```python
from build123d import *

# Parameters (mm, degrees)
F0_W     = 55.8
F0_H     = 27.9
F0_R     = 1.5
F0_R_2   = 3
F1_DEPTH = 4
F2_R     = 13.94999


# Not quite as in the source:
# - a fillet or chamfer is up to 0.001 mm smaller than in the source, because OpenCascade refuses the exact size


with BuildPart() as f1:
    # F0 (on Top) → F1 (new body)
    with BuildSketch(Plane.XY):
        with Locations((-27.9, 13.95)):
            Rectangle(F0_W, F0_H)
        with Locations((-19.6068542495, 8.2931457505)):
            Circle(F0_R, mode=Mode.SUBTRACT)
        with Locations((-7.2324855787, 7.2324855787)):
            Circle(F0_R, mode=Mode.SUBTRACT)
        with Locations((-20.6675144213, 20.6675144213)):
            Circle(F0_R, mode=Mode.SUBTRACT)
        with Locations((-13.95, 13.95)):
            Circle(F0_R_2, mode=Mode.SUBTRACT)
        with Locations((-8.2931457505, 19.6068542495)):
            Circle(F0_R, mode=Mode.SUBTRACT)
    extrude(amount=F1_DEPTH)

    # F2 (radius 13.95 in the source; OpenCascade refuses exactly that, so slightly less here)
    f2_edges = [f1.edges().sort_by_distance(p)[0] for p in [
        (0, 27.9, 2),
        (0, 0, 2),
    ]]
    fillet(f2_edges, radius=F2_R)


solid = f1.part
```
Geometry: final body of the model. Coordinates: model frame, mm. Coordinates: 2 decimals unless noted, no trailing zeros. Order: outer loops, then holes, each group sorted by start corner. A loop starts at its lowest first (then second) coordinate and runs counter-clockwise, first axis right, second up. Notation, with made-up numbers: (55, 14) - (109, 14) arc R19 ccw to (109, 42) - close; hole circle Ø2 at (31.25, -1.5). An arc over 180 degrees is marked (long way). Return JSON: item names as keys, results as strings. Group by question number.
1. Pull-direction query (X, two-part tool) for faces 1 (the face through (-35, 27.9, 2)), 2 (the face through (-55.8, 14, 2)), 3 (the face through (-22.166, 20.733, 1.972)), 4 (the face through (-4.195, 23.922, 2.028)); classes: pulls with the +X half, pulls with the -X half, needs draft (parallel to the pull), parting line crosses it, or undercut.
2. Pin query (flat end, axial travel): pin 1 (2 mm diameter, centred on x = -9.5, z = 0.5, fed in from -Y). Return the tip coordinate at first contact, or that it passes through.
3. Material intervals for line 1 along X through (y, z) = (20.75, 2.3); line 2 along Y through (x, z) = (-13.95, 2.45); line 3 along X through (y, z) = (12, 3.25), sorted ascending. Write a range as [from, to].
4. Cut plane B-B (y = 16). Output: boundary loops of the cut face in (x, z).
5. Cut plane A-A (z = 0.95). Count the separate pieces of the cut face and the enclosed holes in it, plus the area to 3 significant figures.
Resolved:
{
 "1": {"face 1": "needs draft", "face 2": "pulls with the -X half", "face 3": "undercut", "face 4": "pulls with the +X half"},
 "2": {"pin 1": "stops at y = 0.43"},
 "3": {"line 1": "x = [-55.8, -22.17], [-19.17, -9.26], [-7.32, -1.77]", "line 2": "y = [0, 10.95], [16.95, 27.9]", "line 3": "x = [-55.8, -16.23], [-11.67, -0.14]"},
 "4": {"outline": "(-55.8, 0) - (-16.14, 0) - (-16.14, 4) - (-55.8, 4) - close; (-11.76, 0) - (-0.15, 0) - (-0.15, 4) - (-11.76, 4) - close"},
 "5": {"separate pieces": "1", "enclosed holes": "5", "area": "1,420 mm²"}
}
